Input: part model. Units: mm. Frame: model coordinates. A direction names the side the tool comes from. Coordinates: 2 decimals unless noted, no trailing zeros. Order: outer loops, then holes, each group sorted by start corner. A loop starts at its lowest first (then second) coordinate and runs counter-clockwise, first axis right, second up. Notation, with made-up numbers: M 85,68 L 115,68 A11 ccw 115,82 Z; hole C 66.5,54 d11. An arc over 180 degrees is marked long. One line per item, written item: value.
```python
from build123d import *

# Parameters (mm, degrees)
F1_DEPTH = 4.445
F2_R     = 1.75
F3_DEPTH = 6.859
F5_DEPTH = 3
F6_SIZE  = 1.27


with BuildPart() as f1:
    # F0 (on Top) → F1 (new body, symmetric)
    with BuildSketch(Plane.XY):
        with BuildLine():
            Line((2.159, 12.446), (-4.699, 12.446))
            Line((-4.699, 12.446), (-4.699, 0))
            ThreePointArc((-4.699, 0), (1.2161906929, -4.5388854577), (4.0694533724, 2.3495))
            ThreePointArc((4.0694533724, 2.3495), (3.0285420147, 2.6284113577), (2.749630657, 1.5875))
            ThreePointArc((2.749630657, 1.5875), (-0.8217504682, -3.0668144985), (-1.5875, 2.749630657))
            Line((-1.5875, 2.749630657), (2.159, 4.9126734405))
            Line((2.159, 4.9126734405), (2.159, 12.446))
        make_face()
    extrude(amount=F1_DEPTH, both=True)

    # F2 (on face) → F3 (cut, through all)
    with BuildSketch(Plane.YZ.offset(2.159)):
        with Locations((8.382, 0)):
            Circle(F2_R)
    extrude(amount=-F3_DEPTH, mode=Mode.SUBTRACT)

    # F4 (on face) → F5 (cut)
    with BuildSketch(Plane.YZ.offset(2.159)):
        Polygon((11.2776, -1.6717754395), (11.2776, 1.6717754395), (8.382, 3.3435508789), (5.4864, 1.6717754395), (5.4864, -1.6717754395), (8.382, -3.3435508789), align=None)
    extrude(amount=-F5_DEPTH, mode=Mode.SUBTRACT)

    # F6
    f6_edges = [f1.edges().sort_by_distance(p)[0] for p in [
        (-1.27, 12.446, -4.445),
        (-1.27, 12.446, 4.445),
    ]]
    chamfer(f6_edges, length=F6_SIZE)


solid = f1.part
```
(1) Ray query, line 1 (Y direction, x = 1, z = 0.5); line 2 (Y direction, x = -2.75, z = -1); line 3 (X direction, y = 6.75, z = 1.5). Return the intervals inside material, ascending. Write a range as from..to.
Data:
line 1: y = -4.59..-3.01, 4.24..5.49, 11.28..12.45
line 2: y = -3.81..-1.59, 1.59..6.95, 9.82..12.45
line 3: x = -4.7..-0.84
(2) Access query for faces 1 (the flat face through (-1, 5, 4.445)), 2 (the flat face through (2.159, 9.5, 3)), 3 (the flat face through (-1, 12.446, 0)), 4 (the flat face through (0.26, 3.816, 0.062)), 5 (the flat face through (0.68, 6.914, -2.496)). Directions: +Z, -Z, +X, -X, +Y, -Y. A direction counts if a zero-diameter tool reaches every point of the face in a straight line with its end or side. Return the directions, or none.
Data:
face 1: +Z, +X, -X, +Y, -Y
face 2: +Z, -Z, +X, +Y
face 3: +Z, -Z, +X, -X, +Y
face 4: +Z, -Z, +X
face 5: +X
(3) First-contact query: pin 1 (4 mm diameter, centred on y = -1, z = -1, fed in from -X); pin 2 (3 mm diameter, centred on y = 7, z = -1, fed in from +X). Flat tips, straight axial feed; report the tip coordinate or a pass-through.
Data:
pin 1: stops at x = -4.7
pin 2: stops at x = 2.16
(4) Cut plane C-C on y = 8. Output: boundary loops of the cut face in (x, z) (3 decimals), plus the area to 3 significant figures.
Data:
outline: M -4.699,-4.445 L 2.159,-4.445 L 2.159,-3.123 L -0.841,-3.123 L -0.841,-1.708 L -4.699,-1.708 Z; M -4.699,1.708 L -0.841,1.708 L -0.841,3.123 L 2.159,3.123 L 2.159,4.445 L -4.699,4.445 Z
area: 29.1 mm2
(5) Cut plane D-D on x = 0. Output: boundary loops of the cut face in (y, z) (3 decimals), plus the area to 3 significant figures.
Data:
outline: M -4.699,-4.445 L -3.175,-4.445 L -3.175,4.445 L -4.699,4.445 Z; M 3.666,-4.445 L 11.176,-4.445 L 12.446,-3.175 L 12.446,3.175 L 11.176,4.445 L 3.666,4.445 Z; hole M 5.486,-1.672 L 8.382,-3.344 L 11.278,-1.672 L 11.278,1.672 L 8.382,3.344 L 5.486,1.672 Z
area: 60.9 mm2
(6) Cut plane A-A on x = 1.25. Output: boundary loops of the cut face in (y, z) (3 decimals).
Data:
outline: M -4.53,-4.445 L -2.919,-4.445 L -2.919,4.445 L -4.53,4.445 Z; M 4.388,-4.445 L 11.176,-4.445 L 12.446,-3.175 L 12.446,3.175 L 11.176,4.445 L 4.388,4.445 Z; hole M 5.486,-1.672 L 8.382,-3.344 L 11.278,-1.672 L 11.278,1.672 L 8.382,3.344 L 5.486,1.672 Z
(7) Draft query along Z for faces 6 (the cylindrical face through (-0.72, -3.092, 0.062)), 7 (the flat face through (-1, 5, -4.445)), 8 (the flat face through (0.68, 9.81, -2.52)), 9 (the flat face through (0.68, 6.954, 2.519)). Return one class per face: released by +Z, released by -Z, zero draft, split by the parting line, or undercut.
Data:
face 6: zero draft
face 7: released by -Z
face 8: undercut
face 9: undercut
